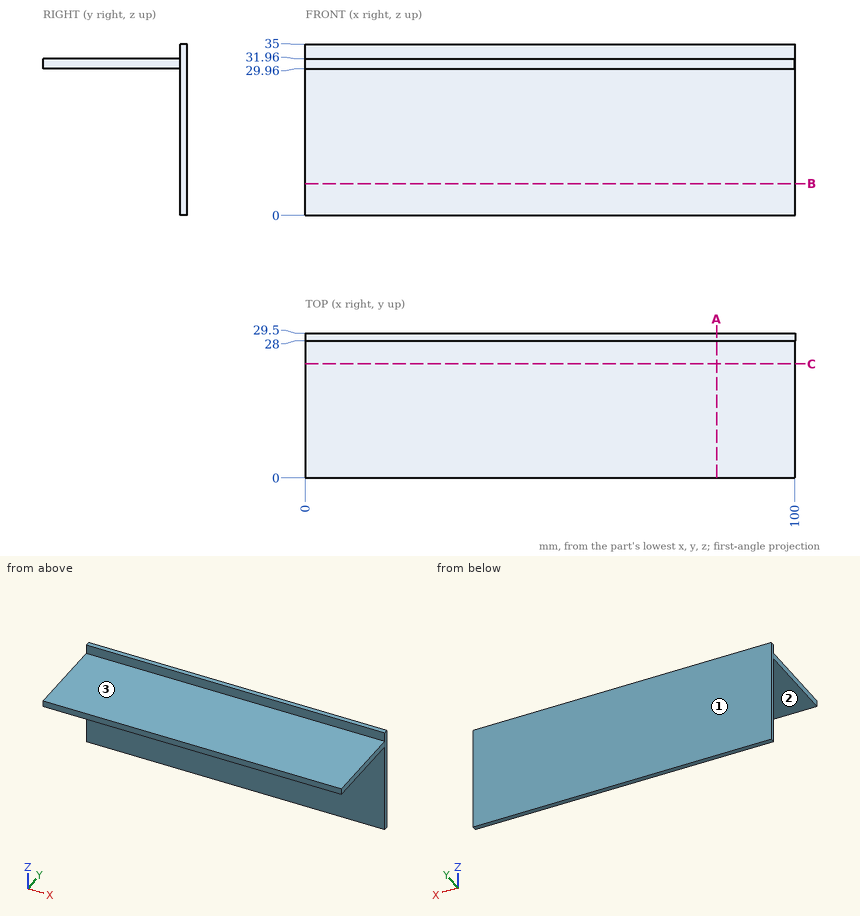
Here's the drawing with two shaded views (mm, measured from the low corner). I have some questions. A direction names the side the tool comes from. Give positions to 0.01 mm unless a question says otherwise; leave off trailing zeros. Loops run counter-clockwise (first coordinate to the right, second up) from the corner with the lowest first, then second, coordinate; pieces in that order, holes last. Notation, with made-up numbers: M -35.75,78.25 L 17.25,78.25 A7 ccw 17.25,90.25 Z; hole C 23,-16 d11. An arc over 180 degrees is marked long. One line per item, written item: value. Start each with the question number.
1) On a 3-axis mill with a long thin cutter (end or side, diameter ignored), from which of +Z, -Z, +X, -X, +Y, -Y can I reach the whole of each face in a straight line? I mean the marked faces 1, 2 and 3. Say none if no direction works.
2) If I drill on line 1 (Z direction, x = 61, y = 16); line 2 (Y direction, x = 66.5, z = 6), over which ranges is the centre line in solid material (lowest first)? Write a range as [from, to].
3) If we section it at A-A, the plane x = 84: Write out the boundary of the cut face in (y, z), and give its area (4 significant figures).
4) If we section it at C-C, the plane y = 23.25: Write out the boundary of the cut face in (x, z), and give its area (3 significant figures).
5) If we section it at B-B, the plane z = 6.5: Write out the boundary of the cut face in (x, y).
6) I'm going to push flat-ended pins straight in: pin 1 (4 mm diameter, centred on x = 49, z = 28.5, fed in from -Y); pin 2 (4 mm diameter, centred on x = 54.5, y = 8.5, fed in from +Z); pin 3 (10 mm diameter, centred on x = 32, y = 13, fed in from -Z). Where does each tip first touch, or does it pass through?
Completed:
1. face 1: +Z, -Z, +X, -X, +Y
1. face 2: -Z, +X, -X, -Y
1. face 3: +Z, +X, -X, -Y
2. line 1: z = [29.96, 31.96]
2. line 2: y = [28, 29.5]
3. outline: M 0,29.96 L 28,29.96 L 28,0 L 29.5,0 L 29.5,35 L 28,35 L 28,31.96 L 0,31.96 Z
3. area: 108.5 mm^2
4. outline: M 0,29.96 L 100,29.96 L 100,31.96 L 0,31.96 Z
4. area: 200 mm^2
5. outline: M 0,28 L 100,28 L 100,29.5 L 0,29.5 Z
6. pin 1: stops at y = 0
6. pin 2: stops at z = 31.96
6. pin 3: stops at z = 29.96
